The model under review builds one solid part; all positions refer to its coordinate system, in mm. A direction names the side the tool comes from. Coordinates: 2 decimals unless noted, no trailing zeros. Loops run counter-clockwise (first coordinate to the right, second up) from the corner with the lowest first, then second, coordinate; pieces in that order, holes last. Notation, with made-up numbers: (65.25, -40) - (83.25, -40) arc R25 cw to (83.25, -24) - close; hole circle Ø1 at (30, 27.25). An arc over 180 degrees is marked (long way). One line per item, written item: value. Start each with the question number.
1. We need section A-A, the plane y = -0.4. Give the boundary of the cut face in (x, z).
2. We need section D-D, the plane x = 0. Give the boundary of the cut face in (y, z), then the cut area to 3 significant figures.
3. Insertion check: P1, Ø1, axis at x = 6, z = 3.5, coming from the +Y side; P2, Ø0.8, axis at x = 5.5, z = 0, coming from the +Y side; P3, Ø0.6, axis at y = -1.5, z = -5, coming from the -X side (3 decimals); P4, Ø0.6, axis at y = -0.5, z = -4.5, coming from the -X side. Each pin has a flat end and moves straight along its axis. Give the tip position at first contact, or say it passes through.
4. We need section B-B, the plane x = 4. Give the boundary of the cut face in (y, z).
5. We need section C-C, the plane z = 1.25. Give the boundary of the cut face in (x, y).
6. For faces 1 (the face through (0, 0.254, 0)), 2 (the face through (3, -3, -4.318)), 3 (the face through (0, 0, 1)), list the 3-axis set-ups (+Z, -Z, +X, -X, +Y, -Y) from which the entire face can be reached by the end or side of a thin tool; tool diameter is ignored.
7. To check wall thickness, follow line 1 (Z direction, x = 0, y = -1.4); line 2 (Y direction, x = 1.5, z = 0); line 3 (Y direction, x = -0.5, z = -3.25). State the ranges of each line that lie inside material, in increasing order.
8. Mouldability with a two-part tool opening along Z and no side actions: class faces 4 (the face through (3, -3, -0.381)), 5 (the face through (-0.291, -3.255, -4.704)), 6 (the face through (3, -3, 5.08)), 7 (the face through (3, -3, -5.08)) as +Z half, -Z half, draft (parallel to the pull), parting line (faces both ways), or undercut.
Autodesk Inventor part; units mm, degrees
ref_plane "to_base_XY" through (0, -0.0254, 0) normal (0, 1, 0) x (1, 0, 0)
ref_plane "to_base_YZ" through (0, -0.0254, 0) normal (1, 0, 0) x (0, 0, -1)
ref_plane "to_base_ZX" through (0, -0.0254, 0) normal (0, 0, -1) x (0, 1, 0)
sketch "Sketch_2" plane through (0, 0, 0) normal (0, 1, 0) x (-1, 0, 0)
  line L0 (2.9257, -5.0719) -> (2.9257, 5.0719)
  arc A0 (2.9257, 5.0719) -> (2.7957, 5.2019) centre (2.7957, 5.0719) ccw
  line L1 (2.7957, 5.2019) -> (-2.7957, 5.2019)
  arc A1 (-2.7957, 5.2019) -> (-2.9257, 5.0719) centre (-2.7957, 5.0719) ccw
  line L2 (-2.9257, 5.0719) -> (-2.9257, -5.0719)
  arc A2 (-2.9257, -5.0719) -> (-2.7957, -5.2019) centre (-2.7957, -5.0719) ccw
  line L3 (-2.7957, -5.2019) -> (2.7957, -5.2019)
  arc A3 (2.7957, -5.2019) -> (2.9257, -5.0719) centre (2.7957, -5.0719) ccw
extrude "Extrusion1" add sketch "Sketch_2" along normal blind 0.254
sketch "Sketch_1" plane through (0, 0, -4.699) normal (0, 0, 1) x (1, 0, 0)
  line L0 (-0.889, 0) -> (-0.889, -1.016)
  line L1 (-0.889, -1.016) -> (-0.635, -1.016)
  line L2 (-0.635, -1.016) -> (-0.635, -2.4384)
  arc A0 (-0.635, -2.4384) -> (0.508, -3.5814) centre (0.508, -2.4384) ccw
  line L3 (0.508, -3.5814) -> (7.6073, -3.5814)
  arc A1 (7.6073, -3.5814) -> (7.6073, -2.3114) centre (7.6073, -2.9464) ccw
  line L4 (7.6073, -2.3114) -> (1.143, -2.3114)
  arc A2 (0.635, -1.8034) -> (1.143, -2.3114) centre (1.143, -1.8034) ccw
  line L5 (0.635, -1.8034) -> (0.635, -1.016)
  line L6 (0.635, -1.016) -> (0.889, -1.016)
  line L7 (0.889, -1.016) -> (0.889, 0)
  line L8 (0.889, 0) -> (-0.889, 0)
extrude "Extrusion2" add sketch "Sketch_1" along normal mid plane 0.762
pattern_linear "Rectangular Pattern1" count 3 spacing 4.699 along (0, 0, 1) of "Extrusion2"
ref_plane "to_base_XY" through (0, -0.0254, 0) normal (0, 1, 0) x (1, 0, 0)
ref_plane "to_base_YZ" through (0, -0.0254, 0) normal (1, 0, 0) x (0, 0, -1)
ref_plane "to_base_ZX" through (0, -0.0254, 0) normal (0, 0, -1) x (0, 1, 0)
properties part number "M201230_terminal_angW"
Findings below:
1. outline: (-0.89, -5.08) - (0.89, -5.08) - (0.89, -4.32) - (-0.89, -4.32) - close; (-0.89, -0.38) - (0.89, -0.38) - (0.89, 0.38) - (-0.89, 0.38) - close; (-0.89, 4.32) - (0.89, 4.32) - (0.89, 5.08) - (-0.89, 5.08) - close
2. outline: (-3.46, -5.08) - (0, -5.08) - (0, -5.2) - (0.25, -5.2) - (0.25, 5.2) - (0, 5.2) - (0, 5.08) - (-3.46, 5.08) - (-3.46, 4.32) - (0, 4.32) - (0, 0.38) - (-3.46, 0.38) - (-3.46, -0.38) - (0, -0.38) - (0, -4.32) - (-3.46, -4.32) - close
2. area: 10.6 mm2
3. P1: through
3. P2: y = -2.31
3. P3: x = -0.635
3. P4: x = -0.89
4. outline: (-3.58, -5.08) - (-2.31, -5.08) - (-2.31, -4.32) - (-3.58, -4.32) - close; (-3.58, -0.38) - (-2.31, -0.38) - (-2.31, 0.38) - (-3.58, 0.38) - close; (-3.58, 4.32) - (-2.31, 4.32) - (-2.31, 5.08) - (-3.58, 5.08) - close
5. outline: (-2.93, 0) - (2.93, 0) - (2.93, 0.25) - (-2.93, 0.25) - close
6. face 1: +Z, -Z, +X, -X, +Y
6. face 2: +X, -X, -Y
6. face 3: none
7. line 1: -5.08 to -4.32, -0.38 to 0.38, 4.32 to 5.08
7. line 2: -3.58 to -2.31, 0 to 0.25
7. line 3: 0 to 0.25
8. face 4: undercut
8. face 5: draft
8. face 6: +Z half
8. face 7: -Z half
